For this review, take the finished solid that the model builds, in its own axes (mm). A direction names the side the tool comes from. Round coordinates to 2 decimals unless told otherwise and drop trailing zeros. Order: outer loops, then holes, each group sorted by start corner. A loop starts at its lowest first (then second) coordinate and runs counter-clockwise, first axis right, second up. Notation, with made-up numbers: M 58.25,0.25 L 87.25,0.25 A28 cw 87.25,26.25 Z; hole C -17.75,23 d3. An arc over 180 degrees is marked long. Put each result on its own line as item: value.
Autodesk Inventor part; units mm, degrees
ref_plane "YZ Plane" through (0, 0, 0) normal (1, 0, 0) x (0, 1, 0)
ref_plane "XZ Plane" through (0, 0, 0) normal (0, 1, 0) x (-1, 0, 0)
ref_plane "XY Plane" through (0, 0, 0) normal (0, 0, 1) x (1, 0, 0)
sketch "Szkic1" plane through (0, 0, 0) normal (0, 1, 0) x (-1, 0, 0)
  line L0 (-8, -90) -> (-52, -90)
  line L1 (-60, -82) -> (-60, 82)
  line L2 (-52, 90) -> (-8, 90)
  line L3 (0, 82) -> (0, -82)
  arc A0 (-8, -90) -> (0, -82) centre (-8, -82) ccw
  arc A1 (-60, -82) -> (-52, -90) centre (-52, -82) ccw
  arc A2 (0, 82) -> (-8, 90) centre (-8, 82) ccw
  arc A3 (-52, 90) -> (-60, 82) centre (-52, 82) ccw
  line L4 (-2.3431, -87.6569) -> (125.3697, -38.6325)
  line L5 (-2.3431, -87.6569) -> (134.4558, -87.6569) construction
  line L6 (-2.3431, 87.6569) -> (125.3697, 38.6325)
  line L7 (-2.3431, 87.6569) -> (134.4558, 87.6569) construction
  line L8 (193.533, -17) -> (224, -17)
  line L9 (224, 17) -> (193.533, 17)
  line L10 (193.533, -17) -> (133.3303, -17)
  line L11 (193.533, 17) -> (133.3303, 17)
  line L12 (224, -17) -> (224, -32.5)
  line L13 (224, 17) -> (224, 32.5)
  line L14 (224, 32.5) -> (138.3184, 32.5)
  line L15 (224, -32.5) -> (138.3184, -32.5)
  arc A4 (133.3303, 17) -> (133.3303, -17) centre (115, 0) ccw
  arc A5 (151.2077, 17) -> (151.2077, -17) centre (115, 0) ccw
  point P0 (0, 0)
  point P1 (-60, 90)
  point P2 (-60, -90)
  point P3 (0, 90)
  point P4 (-30, 0)
  point P5 (125.3697, 38.6325)
  dimension "d0" = 60
  dimension "d1" = 180
  dimension "d2" = 8
  dimension "d5" = 21
  dimension "d6" = 21
  dimension "d9" = 15.5
  dimension "d10" = 15.5
extrude "Wyciągnięcie proste1" add sketch "Szkic1" along normal blind 100
sketch "Szkic2" plane through (0, 100, 0) normal (0, 1, 0) x (1, 0, 0)
  line L0 (8, -90) -> (52, -90)
  line L1 (60, -82) -> (60, 82)
  line L2 (52, 90) -> (8, 90)
  line L3 (0, 82) -> (0, -82)
  arc A0 (0, -82) -> (8, -90) centre (8, -82) ccw
  arc A1 (8, 90) -> (0, 82) centre (8, 82) ccw
  arc A2 (60, 82) -> (52, 90) centre (52, 82) ccw
  arc A3 (52, -90) -> (60, -82) centre (52, -82) ccw
  point P0 (0, 0)
  dimension "d13" = 8
extrude "Wyciągnięcie proste2" cut sketch "Szkic2" against normal blind 64
sketch "Szkic3" plane through (0, 100, 0) normal (0, 1, 0) x (1, 0, 0)
  arc A0 (-138.3184, -32.5) -> (-125.3697, -38.6325) centre (-115, 0) ccw
  arc A1 (-125.3697, 38.6325) -> (-138.3184, 32.5) centre (-115, 0) ccw
  arc A2 (-138.3184, -32.5) -> (-138.3184, 32.5) centre (-115, 0) ccw
  line L0 (-125.3697, -38.6325) -> (2.3431, -87.6569)
  line L1 (-125.3697, -38.6325) -> (2.3431, -87.6569)
  line L2 (2.3431, 87.6569) -> (-125.3697, 38.6325)
  line L3 (-125.3697, 38.6325) -> (2.3431, 87.6569)
  line L4 (0, -82) -> (0, 82)
  line L5 (0, -82) -> (0, 82)
  arc A3 (0, -82) -> (2.3431, -87.6569) centre (8, -82) ccw
  arc A4 (0, -82) -> (2.3431, -87.6569) centre (8, -82) ccw
  arc A5 (8, 90) -> (2.3431, 87.6569) centre (8, 82) ccw
  arc A6 (8, 90) -> (0, 82) centre (8, 82) ccw
  point P0 (0, 0)
  point P1 (-125.3697, 38.6325)
  point P2 (-125.3697, -38.6325)
extrude "Wyciągnięcie proste3" cut sketch "Szkic3" against normal blind 74
sketch "Szkic4" plane through (0, 0, 0) normal (0, -1, 0) x (1, 0, 0)
  line L0 (-224, 32.5) -> (-138.3184, 32.5)
  line L1 (-224, 32.5) -> (-138.3184, 32.5)
  line L2 (-224, 17) -> (-224, 32.5)
  line L3 (-224, 32.5) -> (-224, 17)
  arc A0 (-125.3697, 38.6325) -> (-138.3184, 32.5) centre (-115, 0) ccw
  arc A1 (-138.3184, 32.5) -> (-151.2077, 17) centre (-115, 0) ccw
  line L4 (-133.3303, 17) -> (-224, 17)
  line L5 (-224, 17) -> (-151.2077, 17)
  arc A2 (-138.3184, -32.5) -> (-125.3697, -38.6325) centre (-115, 0) ccw
  arc A3 (-151.2077, -17) -> (-137.5648, -33.0277) centre (-115, 0) ccw
  line L6 (-224, -17) -> (-133.3303, -17)
  line L7 (-151.2077, -17) -> (-224, -17)
  line L8 (-224, -32.5) -> (-224, -17)
  line L9 (-224, -17) -> (-224, -32.5)
  line L10 (-224, -32.5) -> (-138.3184, -32.5)
  point P0 (0, 0)
  point P1 (-138.3184, -32.5)
  dimension "d18" = 40
extrude "Wyciągnięcie proste4" cut sketch "Szkic4" against normal blind 26
sketch "Szkic5" plane through (0, 100, 0) normal (0, 1, 0) x (1, 0, 0)
  arc A0 (-138.3184, 32.5) -> (-151.2077, 17) centre (-115, 0) ccw
  arc A1 (-138.3184, 32.5) -> (-151.2077, 17) centre (-115, 0) ccw
  arc A2 (-151.2077, -17) -> (-125.3697, -38.6325) centre (-115, 0) ccw
  line L0 (-224, -32.5) -> (-138.3184, -32.5)
  arc A3 (-151.2077, -17) -> (-138.3184, -32.5) centre (-115, 0) ccw
  line L1 (-138.3184, 32.5) -> (-224, 32.5)
  line L2 (-138.3184, 32.5) -> (-224, 32.5)
  line L3 (-224, 32.5) -> (-224, 17)
  line L4 (-224, 32.5) -> (-224, 17)
  line L5 (-224, 17) -> (-151.2077, 17)
  line L6 (-133.3303, -17) -> (-224, -17)
  line L7 (-151.2077, -17) -> (-224, -17)
  line L8 (-224, -17) -> (-224, -32.5)
  line L9 (-224, -17) -> (-224, -32.5)
  line L10 (-224, -32.5) -> (-138.3184, -32.5)
  point P0 (0, 0)
extrude "Wyciągnięcie proste5" cut sketch "Szkic5" against normal blind 34
sketch "Szkic6" plane through (-224, 26, 32.5) normal (0, 0, 1) x (1, 0, 0)
  point P0 (224, -26)
sketch "Szkic7" plane through (0, 36, 0) normal (0, 1, 0) x (1, 0, 0)
  line L0 (8, 90) -> (52, 90)
  line L1 (60, 82) -> (60, -82)
  point P0 (0, 0)
  point P1 (28, 55)
  point P2 (30, 90)
  point P3 (28, -55)
  dimension "d23" = 35
  dimension "d24" = 32
sketch "Szkic8" plane through (0, 26, 0) normal (0, 1, 0) x (1, 0, 0)
  point P0 (0, 0)
  point P1 (44, 0)
  point P2 (44, 0)
  point P3 (-44, 0)
hole "Otwór1" at (-44, 26, 0) direction (0, -1, 0) diameter 24 end through all
hole "Otwór2" at (28, 36, -55) at (28, 36, 55) direction (0, -1, 0) diameter 25 end through all counterbore diameter 35 counterbore depth 20
sketch "Szkic9" plane through (-224, 26, 32.5) normal (0, 0, 1) x (1, 0, 0)
  point P0 (224, -26)
sketch "Szkic10" plane through (-224, 26, 32.5) normal (0, 0, 1) x (1, 0, 0)
  point P0 (224, -26)
  point P1 (20, 20)
hole "Otwór3" at (-204, 46, 32.5) direction (0, 0, -1) diameter 24 end through all
full round fillet "Zaokrąglenie pełne1" first side at (-199.7359, 66, -22.1667) centre faces at (-224, 39.3333, -27.3333) second side at (-199.7359, 26, -22.1667)
full round fillet "Zaokrąglenie pełne2" first side at (-199.7359, 66, 22.1667) centre faces at (-224, 39.3333, 22.1667) second side at (-199.7359, 26, 22.1667)
(1) Add section D-D on x = -110.5. Give the boundary of the cut face in (y, z), then the cut area to 3 significant figures.
A:
outline: M 0,-44.34 L 26,-44.34 L 26,-39.75 L 100,-39.75 L 100,-24.59 L 0,-24.59 Z; M 0,24.59 L 100,24.59 L 100,39.75 L 26,39.75 L 26,44.34 L 0,44.34 Z
area: 3,270 mm2
(2) To check wall thickness, follow L1, parallel to Z at x = 28, y = 5; L2, parallel to Y at x = -204, z = -28.75; L3, parallel to X at y = 32, z = -55. State the ranges of each line that lie inside material, in increasing order.
A:
L1: z = -90 to -67.5, -42.5 to 42.5, 67.5 to 90
L2: y = 26 to 34, 58 to 66
L3: x = 0 to 10.5, 45.5 to 60
(3) Add section B-B on z = 0. Give the boundary of the cut face in (x, y), then the cut area to 3 significant figures.
A:
outline: M -90,0 L -56,0 L -56,26 L -75,26 L -75,100 L -90,100 Z; M -32,0 L 60,0 L 60,36 L 0,36 L 0,26 L -32,26 Z
area: 4,990 mm2
(4) Insertion check: pin 1 Ø4.5 at (x, z) = (-170, -26.5) entering from +Y; pin 2 Ø1.5 at (x, z) = (2, -1) entering from +Y; pin 3 Ø8 at (x, z) = (-164.5, -28) entering from -Y. Each pin has a flat end and moves straight along its axis. Give the tip position at first contact, or say it passes through.
A:
pin 1: stops at y = 66
pin 2: stops at y = 36
pin 3: stops at y = 26
(5) For faces 4 (the face through (-172, 46, -32.5)), 5 (the face through (22.74, 25.86, -38.31)), 6 (the face through (4.54, 21.748, -89.213)), 7 (the face through (0, 31, 1)), list the 3-axis set-ups (+Z, -Z, +X, -X, +Y, -Y) from which the entire face can be reached by the end or side of a thin tool; tool diameter is ignored.
A:
face 4: -Z, -X, +Y, -Y
face 5: +Y
face 6: -Z, -X, +Y
face 7: +Z, -Z, +Y
(6) Draft analysis for pull direction X (two halves, no side actions). For faces 1 (the face through (30, 18, -90)), 2 (the face through (-60.619, 12.818, -63.488)), 3 (the face through (27.45, 7.888, -67.488)), state which applies: released by +X, released by -X, zero draft, split by the parting line, or undercut.
A:
face 1: zero draft
face 2: released by -X
face 3: undercut
(7) Add section A-A on x = -188. Give the boundary of the cut face in (y, z).
A:
outline: M 26,-32.5 L 66,-32.5 L 66,-17 L 26,-17 Z; M 26,17 L 66,17 L 66,32.5 L 26,32.5 Z
(8) Add section C-C on y = 87. Give the boundary of the cut face in (x, z).
A:
outline: M -151.21,-17 A40 ccw -138.32,-32.5 A40 ccw long -138.32,32.5 A40 ccw -151.21,17 L -133.33,17 A25 cw long -133.33,-17 Z
